Answer from the drawing. Dimensions are ordinates in mm from the lowest x, y and z of the part. A direction names the side the tool comes from. Coordinates: 2 decimals unless noted, no trailing zeros. Write each loop counter-clockwise with the first axis right and the second up, starting at its lowest first coordinate (ties: lowest second). Pieces come first, ordered by that corner, then holes. Notation, with made-up numbers: M 72.5,-4.5 L 86.5,-4.5 A24 cw 86.5,7.5 Z; hole C 2.5,-15.5 d9. An arc over 180 degrees is marked long. Put each result on its own line as item: value. Start each with the question number.
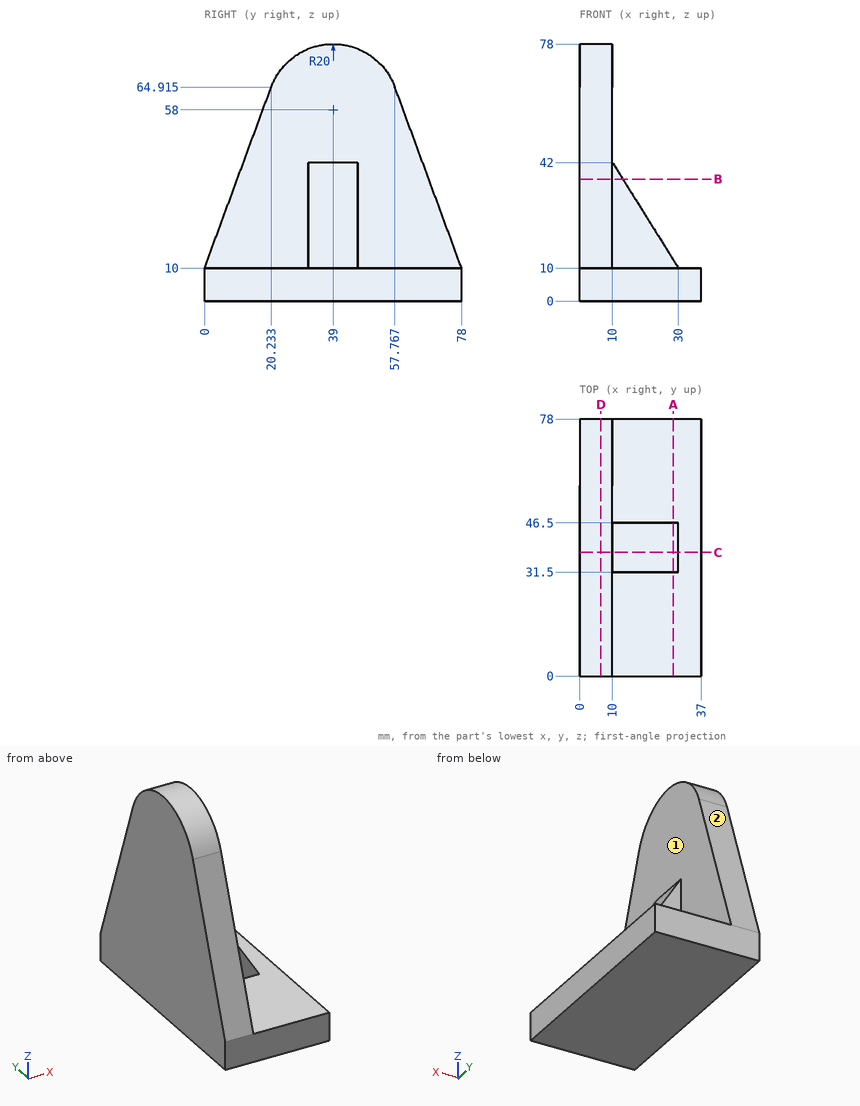
1) Given pin 1 Ø6 at (x, z) = (23, 25.5) entering from +Y; pin 2 Ø8 at (x, z) = (15.5, 22) entering from -Y, each flat-ended and moving along its own axis, determine where each tip first touches the part or whether it passes through.
2) For the marked faces 1 and 2, determine the directions among +Z, -Z, +X, -X, +Y, -Y from which every point of the face is accessible in a straight line to the end or side of a thin tool.
3) Straight lines are drawn through the part: probe 1 along X at (y, z) = (28.5, 74.5); probe 2 along Y at (x, z) = (21.5, 13). For each, find the intervals that lie inside material, in ascending order.
4) A cutting plane is placed at C-C on y = 37.5. Write down the section's boundary in (x, z), then the cut area to 3 significant figures.
5) A cutting plane is placed at D-D on x = 6.5. Write down the section's boundary in (y, z) (1 decimal), then the cut area to 3 significant figures.
6) A cutting plane is placed at A-A on x = 28.5. Write down the section's boundary in (y, z).
7) A cutting plane is placed at B-B on z = 37. Write down the section's boundary in (x, y) (1 decimal), then the cut area to 3 significant figures.
Answers follow:
1. pin 1: stops at y = 46.5
1. pin 2: stops at y = 31.5
2. face 1: +Z, +X
2. face 2: +Z, +X, -X, +Y
3. probe 1: x = 0 to 10
3. probe 2: y = 31.5 to 46.5
4. outline: M 0,0 L 37,0 L 37,10 L 30,10 L 10,42 L 10,77.94 L 0,77.94 Z
4. area: 1,370 mm²
5. outline: M 0,0 L 78,0 L 78,10 L 57.8,64.9 A20 ccw 20.2,64.9 L 0,10 Z
5. area: 4,310 mm²
6. outline: M 0,0 L 78,0 L 78,10 L 46.5,10 L 46.5,12.4 L 31.5,12.4 L 31.5,10 L 0,10 Z
7. outline: M 0,9.9 L 10,9.9 L 10,31.5 L 13.1,31.5 L 13.1,46.5 L 10,46.5 L 10,68.1 L 0,68.1 Z
7. area: 628 mm²
